Input: part model. Units: mm. Frame: model coordinates. Face numbers are marked on the shaded views. A direction names the side the tool comes from. Round coordinates to 2 decimals unless told otherwise and drop trailing zeros. Loops run counter-clockwise (first coordinate to the right, second up) from the corner with the lowest first, then second, coordinate; pieces in that order, holes last. Notation, with made-up numbers: M 13,-24 L 72,-24 A28 cw 72,-5 Z; hole C -23.5,-24.75 d4. An arc over 180 degrees is marked long. Put each result on its own line as item: value. Start each with the question number.
1) Section A-A on y = 32. Output: boundary loops of the cut face in (x, z) (3 decimals), plus the area to 3 significant figures.
2) Reachability of the marked faces 1, 2 and 3 from +Z, -Z, +X, -X, +Y, -Y: full face, straight path, thin tool, end or side. Return the list, or none.
3) Pin query (flat end, axial travel): pin 1 (4 mm diameter, centred on y = 11, z = -2.5, fed in from +X); pin 2 (5 mm diameter, centred on y = 35.56, z = 0, fed in from -X); pin 3 (1 mm diameter, centred on x = -3.5, z = 4.5, fed in from +Y). Return the tip coordinate at first contact, or that it passes through.
4) Line query: probe 1 along Y at (x, z) = (0.3, 0); probe 2 along Y at (x, z) = (1.5, -1.75); probe 3 along X at (y, z) = (20.5, -0.25). Output: solid intervals per line, ascending.
5) Section B-B on y = -3. Output: boundary loops of the cut face in (x, z).
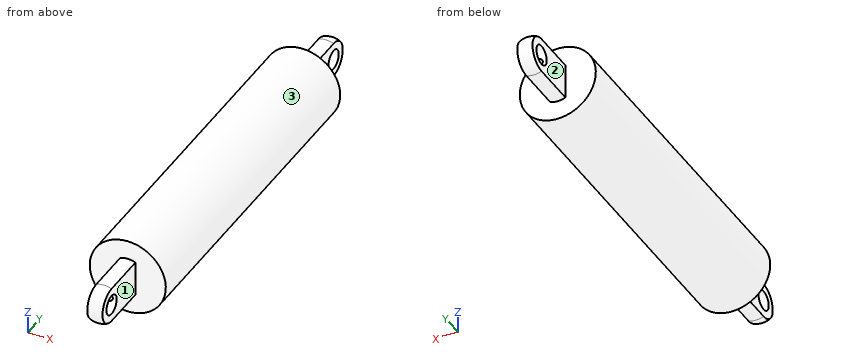
from build123d import *

# Parameters (mm, degrees)
CUT_EXTRUDE2_DEPTH = 68.277043819
SKETCH4_R          = 1.627
CUT_EXTRUDE3_DEPTH = 40.984836188


with BuildPart() as part:
    # Sketch1 → Revolve-Thin1 (revolve)
    with BuildSketch(Plane(origin=(0, 0, 0), x_dir=(0, 0, -1), z_dir=(1, 0, 0))):
        with BuildLine():
            ThreePointArc((0, 38.735), (-2.24506403, 37.80506403), (-3.175, 35.56))
            Line((-3.175, 35.56), (-3.175, 27.94))
            Line((-3.175, 27.94), (-6.35, 27.94))
            Line((-6.35, 27.94), (-6.35, -27.94))
            Line((-6.35, -27.94), (-3.175, -27.94))
            Line((-3.175, -27.94), (-3.175, -35.56))
            ThreePointArc((-3.175, -35.56), (-2.24506403, -37.80506403), (0, -38.735))
            Line((0, -38.735), (0, -36.195))
            ThreePointArc((0, -36.195), (-0.449012806, -36.009012806), (-0.635, -35.56))
            Line((-0.635, -35.56), (-0.635, -25.4))
            Line((-0.635, -25.4), (-3.81, -25.4))
            Line((-3.81, -25.4), (-3.81, 25.4))
            Line((-3.81, 25.4), (-0.635, 25.4))
            Line((-0.635, 25.4), (-0.635, 35.56))
            ThreePointArc((-0.635, 35.56), (-0.449012806, 36.009012806), (0, 36.195))
            Line((0, 36.195), (0, 38.735))
        make_face()
    revolve(axis=Axis((0, 35.56, 0), (0, -1, 0)))

    # Sketch3 → Cut-Extrude2 (cut, through all)
    with BuildSketch(Plane(origin=(0, 27.94, 0), x_dir=(1, 0, 0), z_dir=(0, 1, 0))):
        with BuildLine():
            ThreePointArc((-1.27, 2.909935566), (-3.175, 0), (-1.27, -2.909935566))
            Line((-1.27, -2.909935566), (-1.27, 2.909935566))
        make_face()
        with BuildLine():
            Line((1.27, 2.909935566), (1.27, -2.909935566))
            ThreePointArc((1.27, -2.909935566), (2.656395584, -1.73901912), (3.175, 0))
            ThreePointArc((3.175, 0), (2.656395584, 1.73901912), (1.27, 2.909935566))
        make_face()
    cut_extrude2 = extrude(amount=CUT_EXTRUDE2_DEPTH, mode=Mode.SUBTRACT)

    # Mirror1: Cut-Extrude2 across plane
    add(cut_extrude2.mirror(Plane.ZX), mode=Mode.SUBTRACT)

    # Sketch4 → Cut-Extrude3 (cut, through all)
    with BuildSketch(Plane(origin=(1.27, 0, 0), x_dir=(0, 0, -1), z_dir=(1, 0, 0))):
        with Locations((0, 35.56)):
            Circle(SKETCH4_R)
        with Locations((0, -35.56)):
            Circle(SKETCH4_R)
    extrude(amount=-CUT_EXTRUDE3_DEPTH, mode=Mode.SUBTRACT)


solid = part.part
Geometry results:
1. outline: M -1.27,-2.91 A3.175 ccw 1.27,-2.91 L 1.27,2.91 A3.175 ccw -1.27,2.91 Z; hole C 0,0 d1.27
1. area: 14.4 mm²
2. face 1: +Z, -Z, +X, -Y
2. face 2: +Z, -Z, -X, +Y
2. face 3: +Y, -Y
3. pin 1: stops at x = 6.33
3. pin 2: stops at x = -1.27
3. pin 3: stops at y = 27.94
4. probe 1: y = -38.72 to -37.19, 37.19 to 38.72
4. probe 2: y = -27.94 to -25.4, 25.4 to 27.94
4. probe 3: x = -6.35 to -3.8, 3.8 to 6.35
5. outline: C 0,0 d12.7; hole C 0,0 d7.62
